from build123d import *

# Parameters (mm, degrees)
SKETCH1_W           = 40.0812
SKETCH1_H           = 20.066
BOSS_EXTRUDE1_DEPTH = 41.7068
SKETCH2_W           = 3.175
SKETCH2_H           = 20.066
BOSS_EXTRUDE2_DEPTH = 7.25
CUT_EXTRUDE1_REACH  = 61.993
SKETCH3_R           = 2.2225
SKETCH4_R           = 3.5687
BOSS_EXTRUDE3_DEPTH = 4.064


with BuildPart() as part:
    # Sketch1 → Boss-Extrude1 (new body)
    with BuildSketch(Plane.XY):
        with Locations((20.0406, 10.033)):
            Rectangle(SKETCH1_W, SKETCH1_H)
    extrude(amount=BOSS_EXTRUDE1_DEPTH)

    # Sketch2 → Boss-Extrude2 (add)
    with BuildSketch(Plane(origin=(40.0812, 0, 0), x_dir=(0, 0, -1), z_dir=(1, 0, 0))):
        with Locations((-29.337, 10.033)):
            Rectangle(SKETCH2_W, SKETCH2_H)
    boss_extrude2 = extrude(amount=BOSS_EXTRUDE2_DEPTH)

    # Mirror1: Boss-Extrude2 across plane
    add(boss_extrude2.mirror(Plane.ZY.offset(-20.0406)))

    # Sketch3 → Cut-Extrude1 (cut, up to next)
    with BuildSketch(Plane.XY.offset(30.9245), mode=Mode.PRIVATE) as cut_extrude1_sk1:
        with Locations((44.5516, 5.1816)):
            Circle(SKETCH3_R)
    cut_extrude1_tool1 = extrude(cut_extrude1_sk1.sketch, amount=-CUT_EXTRUDE1_REACH, mode=Mode.PRIVATE) & part.part
    # Sketch3 → Cut-Extrude1 (cut, up to next)
    with BuildSketch(Plane.XY.offset(30.9245), mode=Mode.PRIVATE) as cut_extrude1_sk2:
        with Locations(Location((-4.4704, 5.1816, 0), (0, 0, 180))):
            Circle(SKETCH3_R)
    cut_extrude1_tool2 = extrude(cut_extrude1_sk2.sketch, amount=-CUT_EXTRUDE1_REACH, mode=Mode.PRIVATE) & part.part
    # Sketch3 → Cut-Extrude1 (cut, up to next)
    with BuildSketch(Plane.XY.offset(30.9245), mode=Mode.PRIVATE) as cut_extrude1_sk3:
        with Locations((-4.4704, 14.8844)):
            Circle(SKETCH3_R)
    cut_extrude1_tool3 = extrude(cut_extrude1_sk3.sketch, amount=-CUT_EXTRUDE1_REACH, mode=Mode.PRIVATE) & part.part
    # Sketch3 → Cut-Extrude1 (cut, up to next)
    with BuildSketch(Plane.XY.offset(30.9245), mode=Mode.PRIVATE) as cut_extrude1_sk4:
        with Locations((44.5516, 14.8844)):
            Circle(SKETCH3_R)
    cut_extrude1_tool4 = extrude(cut_extrude1_sk4.sketch, amount=-CUT_EXTRUDE1_REACH, mode=Mode.PRIVATE) & part.part
    add(cut_extrude1_tool1.solids().sort_by_distance((44.5516, 5.1816, 30.9245))[0], mode=Mode.SUBTRACT)
    add(cut_extrude1_tool2.solids().sort_by_distance((-4.4704, 5.1816, 30.9245))[0], mode=Mode.SUBTRACT)
    add(cut_extrude1_tool3.solids().sort_by_distance((-4.4704, 14.8844, 30.9245))[0], mode=Mode.SUBTRACT)
    add(cut_extrude1_tool4.solids().sort_by_distance((44.5516, 14.8844, 30.9245))[0], mode=Mode.SUBTRACT)

    # Sketch4 → Boss-Extrude3 (add)
    with BuildSketch(Plane.XY.offset(41.7068)):
        with Locations(Location((30.1244, 10.033, 0), (0, 0, 180))):
            Circle(SKETCH4_R)
    extrude(amount=BOSS_EXTRUDE3_DEPTH)


solid = part.part
Geometry: final body of the model. Coordinates: model frame, mm. A direction names the side the tool comes from. Round coordinates to 2 decimals unless told otherwise and drop trailing zeros. Write each loop counter-clockwise with the first axis right and the second up, starting at its lowest first coordinate (ties: lowest second). Pieces come first, ordered by that corner, then holes. Notation, with made-up numbers: M 65,50.25 L 72,50.25 A21 cw 72,85.25 Z; hole C 27,28.25 d1. An arc over 180 degrees is marked long. Write item = value, one per line.
Item 1: Material intervals for line 1 along Z through (x, y) = (19.5, 13); line 2 along Z through (x, y) = (-2.5, 13); line 3 along X through (y, z) = (4.75, 8), sorted ascending. Write a range as [from, to].
Findings:
line_1 = [0, 41.71]
line_2 = [27.75, 30.92]
line_3 = [0, 40.08]
Item 2: Access query for faces 1 (the face through (-4, 10, 27.75)), 2 (the face through (40.081, 10, 36)), 3 (the face through (0, 10, 36)). Directions: +Z, -Z, +X, -X, +Y, -Y. A direction counts if a zero-diameter tool reaches every point of the face in a straight line with its end or side. Return the directions, or none.
Findings:
face_1 = -Z, -X, +Y, -Y
face_2 = +Z, +X, +Y, -Y
face_3 = +Z, -X, +Y, -Y
Item 3: Section query B-B on x = 29. Return loops of the section in (y, z).
Findings:
outline = M 0,0 L 20.07,0 L 20.07,41.71 L 13.42,41.71 L 13.42,45.77 L 6.65,45.77 L 6.65,41.71 L 0,41.71 Z
Item 4: Pull-direction query (Y, two-part tool) for faces 4 (the face through (40.081, 10, 14)), 5 (the face through (20, 0, 21)), 6 (the face through (42.33, 14.98, 29.36)), 7 (the face through (28.21, 7.02, 43.71)); classes: pulls with the +Y half, pulls with the -Y half, needs draft (parallel to the pull), parting line crosses it, or undercut.
Findings:
face_4 = needs draft
face_5 = pulls with the -Y half
face_6 = undercut
face_7 = parting line crosses it
Item 5: Section query C-C on y = 2. Return loops of the section in (x, z), then the cut area to 3 significant figures.
Findings:
outline = M -7.25,27.75 L 0,27.75 L 0,0 L 40.08,0 L 40.08,27.75 L 47.33,27.75 L 47.33,30.92 L 40.08,30.92 L 40.08,41.71 L 0,41.71 L 0,30.92 L -7.25,30.92 Z
area = 1,720 mm^2
Item 6: Pin query (flat end, axial travel): P1, Ø2, axis at x = -3, y = 14, coming from the +Z side; P2, Ø4, axis at x = 44.55, y = 5.18, coming from the +Z side; P3, Ø10, axis at y = 7, z = 36, coming from the -X side; P4, Ø10, axis at x = 12.5, y = 6.5, coming from the +Z side. Return the tip coordinate at first contact, or that it passes through.
Findings:
P1 = 30.92
P2 = through
P3 = 0
P4 = 41.71
Item 7: Section query D-D on z = 7. Return loops of the section in (x, y).
Findings:
outline = M 0,0 L 40.08,0 L 40.08,20.07 L 0,20.07 Z
Item 8: Section query A-A on y = 16. Return loops of the section in (x, z).
Findings:
outline = M -7.25,27.75 L -6.39,27.75 L -6.39,30.92 L -7.25,30.92 Z; M -2.55,27.75 L 0,27.75 L 0,0 L 40.08,0 L 40.08,27.75 L 42.63,27.75 L 42.63,30.92 L 40.08,30.92 L 40.08,41.71 L 0,41.71 L 0,30.92 L -2.55,30.92 Z; M 46.47,27.75 L 47.33,27.75 L 47.33,30.92 L 46.47,30.92 Z
